Model file for the job. Use its own axes, mm. A direction names the side the tool comes from. Give positions to 0.01 mm unless a question says otherwise; leave off trailing zeros. Order: outer loops, then holes, each group sorted by start corner. A loop starts at its lowest first (then second) coordinate and runs counter-clockwise, first axis right, second up. Notation, with made-up numbers: (72, 54.25) - (122, 54.25) arc R17 cw to (122, 74.25) - close; hole circle Ø5 at (67, -26.75). An arc over 180 degrees is marked (long way). Return JSON: item names as keys, results as strings. Group by question number.
from build123d import *

# Parameters (mm, degrees)
SKETCH2_W                    = 170
SKETCH2_H                    = 15
BASE_FLANGE1_DEPTH           = 0.5
EDGE_FLANGE1_STRIP_W         = 3.4732
EDGE_FLANGE1_STRIP_H         = 0.5
EDGE_FLANGE1_STRIP_CUT_DEPTH = 170
EDGE_FLANGE1_DEPTH           = 170
M4_CLEARANCE_HOLE1_D         = 4.8
SKETCH14_W                   = 10.5
SKETCH14_H                   = 120
CUT_EXTRUDE1_DEPTH           = 90.945817023
BREAK_CORNER1_START          = 7.5
BREAK_CORNER1_DEPTH          = 0.5
BREAK_CORNER1_START_2        = -0.5
BREAK_CORNER1_2_DEPTH        = 0.5
BREAK_CORNER2_START          = 7.5
BREAK_CORNER2_DEPTH          = 0.5
M4_CLEARANCE_HOLE2_D         = 4.8


# Read off the part's stored shape, not the designer's step: Break-Corner1, Break-Corner2
# Sheet-metal steps are written as plain solids
with BuildPart() as part:
    # Sketch2 → Base-Flange1 (new body)
    with BuildSketch(Plane(origin=(0, 0, 0), x_dir=(0, 0, -1), z_dir=(1, 0, 0))):
        Rectangle(SKETCH2_W, SKETCH2_H)
    extrude(amount=-BASE_FLANGE1_DEPTH)

    # Edge-Flange1 strip (across the edge) → Edge-Flange1 strip cut (cut)
    with BuildSketch(Plane(origin=(0, 7.5, -85), x_dir=(0, -1, 0), z_dir=(0, 0, 1))):
        with Locations((-1, -0.25)):
            Rectangle(EDGE_FLANGE1_STRIP_W, EDGE_FLANGE1_STRIP_H)
    extrude(amount=EDGE_FLANGE1_STRIP_CUT_DEPTH, mode=Mode.SUBTRACT)

    # Edge-Flange1 section (across the edge) → Edge-Flange1 (add)
    with BuildSketch(Plane(origin=(0, 7.5, -85), x_dir=(0, -1, 0), z_dir=(0, 0, 1))):
        with BuildLine():
            Line((-0.5, 0.7366), (-0.5, 25))
            Line((-0.5, 25), (0, 25))
            Line((0, 25), (0, 0.7366))
            ThreePointArc((0, 0.7366), (0.215745145, 0.215745145), (0.7366, 0))
            Line((0.7366, 0), (0.7366, -0.5))
            ThreePointArc((0.7366, -0.5), (-0.137808246, -0.137808246), (-0.5, 0.7366))
        make_face()
    extrude(amount=EDGE_FLANGE1_DEPTH)

    # M4 Clearance Hole1 (through all)
    with Locations(Plane(origin=(0, 8, 0), x_dir=(1, 0, 0), z_dir=(0, 1, 0))):
        with Locations((14.5, 75), (14.5, -75)):
            Hole(M4_CLEARANCE_HOLE1_D / 2)

    # Sketch14 → Cut-Extrude1 (cut, through all)
    with BuildSketch(Plane(origin=(0, 8, 0), x_dir=(1, 0, 0), z_dir=(0, 1, 0))):
        with Locations((19.75, 0)):
            Rectangle(SKETCH14_W, SKETCH14_H)
    extrude(amount=-CUT_EXTRUDE1_DEPTH, mode=Mode.SUBTRACT)

    # Break-Corner1 outline → Break-Corner1 (cut)
    with BuildSketch(Plane(origin=(0, 0, 0), x_dir=(1, 0, 0), z_dir=(0, 1, 0)).offset(BREAK_CORNER1_START)):
        with BuildLine():
            Line((25, -85), (25, -80))
            ThreePointArc((25, -80), (23.535533906, -83.535533906), (20, -85))
            Line((20, -85), (25, -85))
        make_face()
        with BuildLine():
            ThreePointArc((20, -60), (23.535533906, -61.464466094), (25, -65))
            Line((25, -65), (25, -60))
            Line((25, -60), (20, -60))
        make_face()
        with BuildLine():
            Line((25, 85), (20, 85))
            ThreePointArc((20, 85), (23.535533906, 83.535533906), (25, 80))
            Line((25, 80), (25, 85))
        make_face()
        with BuildLine():
            Line((25, 60), (25, 65))
            ThreePointArc((25, 65), (23.535533906, 61.464466094), (20, 60))
            Line((20, 60), (25, 60))
        make_face()
    extrude(amount=BREAK_CORNER1_DEPTH, mode=Mode.SUBTRACT)

    # Break-Corner1 2 outline → Break-Corner1 2 (cut)
    with BuildSketch(Plane.YZ.offset(BREAK_CORNER1_START_2)):
        with BuildLine():
            Line((-7.5, 85), (-7.5, 80))
            ThreePointArc((-7.5, 80), (-6.035533906, 83.535533906), (-2.5, 85))
            Line((-2.5, 85), (-7.5, 85))
        make_face()
        with BuildLine():
            ThreePointArc((-2.5, -85), (-6.035533906, -83.535533906), (-7.5, -80))
            Line((-7.5, -80), (-7.5, -85))
            Line((-7.5, -85), (-2.5, -85))
        make_face()
    extrude(amount=BREAK_CORNER1_2_DEPTH, mode=Mode.SUBTRACT)

    # Break-Corner2 outline → Break-Corner2 (add)
    with BuildSketch(Plane(origin=(0, 0, 0), x_dir=(1, 0, 0), z_dir=(0, 1, 0)).offset(BREAK_CORNER2_START)):
        with BuildLine():
            Line((14.5, 60), (14.5, 55))
            ThreePointArc((14.5, 55), (15.964466094, 58.535533906), (19.5, 60))
            Line((19.5, 60), (14.5, 60))
        make_face()
        with BuildLine():
            ThreePointArc((19.5, -60), (15.964466094, -58.535533906), (14.5, -55))
            Line((14.5, -55), (14.5, -60))
            Line((14.5, -60), (19.5, -60))
        make_face()
    extrude(amount=BREAK_CORNER2_DEPTH)

    # M4 Clearance Hole2 (through all)
    with Locations(Plane(origin=(0, 0, 0), x_dir=(0, 0, -1), z_dir=(1, 0, 0))):
        with Locations((-60, 0), (0, 0), (60, 0)):
            Hole(M4_CLEARANCE_HOLE2_D / 2)


solid = part.part
(1) Drop a flat-ended pin along its axis: pin 1 Ø6 at (y, z) = (0, 0) entering from +X. Give the stop position or say it passes through.
(2) Slice it at D-D (x = 7). Give the cut face in (y, z).
(3) Drill centre lines: L1, parallel to X at y = 5.5, z = -24; L2, parallel to Y at x = 10.75, z = 22; L3, parallel to Y at x = -0.3, z = 60. Where is each one in solid material? Low to high.
(4) Slice it at C-C (z = -12.5). Give the cut face in (x, y), and give its area (3 significant figures).
(5) 3-axis set-ups, long thin cutter, end or side, ignore diameter. For faces 1 (the face through (10, 7.5, -1)), 2 (the face through (15.93, 7.75, -58.5)), 3 (the face through (-0.5, -3, 1)): which of +Z, -Z, +X, -X, +Y, -Y reach the whole face in a straight line?
(6) Slice it at A-A (z = 75). Give the cut face in (x, y).
(7) Slice it at B-B (y = 0). Give the cut face in (x, z), and give its area (3 significant figures).
(8) Pull direction X, two halves, no side cores. Call faces 4 (the face through (-0.254, -0.919, -57.783)), 5 (the face through (0, -3, 1)), 6 (the face through (14.81, 7.75, -77.38)): released by +X, released by -X, zero draft, split by the parting line, or undercut.
Result set:
{
 "1": {"pin 1": "stops at x = 0"},
 "2": {"outline": "(7.5, -85) - (8, -85) - (8, 85) - (7.5, 85) - close"},
 "3": {"L1": "x = -0.5 to 0", "L2": "y = 7.5 to 8", "L3": "y = -7.5 to -2.4, 2.4 to 7.44"},
 "4": {"outline": "(-0.5, -7.5) - (0, -7.5) - (0, 6.76) arc R0.74 cw to (0.74, 7.5) - (14.5, 7.5) - (14.5, 8) - (0.74, 8) arc R1.24 ccw to (-0.5, 6.76) - close", "area": "14.8 mm²"},
 "5": {"face 1": "+Z, -Z, +X, -Y", "face 2": "+X, +Y, -Y", "face 3": "+Z, -Z, -X, +Y, -Y"},
 "6": {"outline": "(-0.5, -7.5) - (0, -7.5) - (0, 6.76) arc R0.74 cw to (0.74, 7.5) - (12.1, 7.5) - (12.1, 8) - (0.74, 8) arc R1.24 ccw to (-0.5, 6.76) - close; (16.9, 7.5) - (25, 7.5) - (25, 8) - (16.9, 8) - close"},
 "7": {"outline": "(-0.5, -85) - (0, -85) - (0, -62.4) - (-0.5, -62.4) - close; (-0.5, -57.6) - (0, -57.6) - (0, -2.4) - (-0.5, -2.4) - close; (-0.5, 2.4) - (0, 2.4) - (0, 57.6) - (-0.5, 57.6) - close; (-0.5, 62.4) - (0, 62.4) - (0, 85) - (-0.5, 85) - close", "area": "77.8 mm²"},
 "8": {"face 4": "zero draft", "face 5": "released by +X", "face 6": "undercut"}
}
